Solid Edge part; units mm, degrees
sketch "Sketch1" plane through (0, 0, 0) normal (0, -1, 0) x (1, 0, 0)
  line L0 (0.9, 0.9) -> (0.9, 2.2249)
  arc A0 (-0.9, 2.2249) -> (0.9, 2.2249) centre (0, 0) cw
  line L1 (-0.9, 0.9) -> (-0.9, 2.2249)
  line L2 (-0.9, 0.9) -> (-2.2249, 0.9)
  line L3 (-0.9, -0.9) -> (-2.2249, -0.9)
  line L4 (-0.9, -0.9) -> (-0.9, -2.2249)
  arc A1 (0.9, -2.2249) -> (-0.9, -2.2249) centre (0, 0) cw
  line L5 (0.9, -0.9) -> (0.9, -2.2249)
  line L6 (0.9, -0.9) -> (2.2249, -0.9)
  arc A2 (2.2249, 0.9) -> (2.2249, -0.9) centre (0, 0) cw
  line L7 (0.9, 0.9) -> (2.2249, 0.9)
  arc A3 (-2.2249, 0.9) -> (-2.2249, -0.9) centre (0, 0) ccw
  line L8 (1.5624, 3.2433) -> (1.8936, 2.4029)
  line L9 (1.8936, 2.4029) -> (2.4029, 1.8936)
  line L10 (3.2433, 1.5624) -> (2.4029, 1.8936)
  arc A4 (3.2433, 1.5624) -> (3.2433, -1.5624) centre (0, 0) cw
  line L11 (2.4029, -1.8936) -> (3.2433, -1.5624)
  line L12 (2.4029, -1.8936) -> (1.8936, -2.4029)
  line L13 (1.5624, -3.2433) -> (1.8936, -2.4029)
  line L14 (-1.5624, -3.2433) -> (-1.8936, -2.4029)
  line L15 (-2.4029, -1.8936) -> (-1.8936, -2.4029)
  line L16 (-3.2433, -1.5624) -> (-2.4029, -1.8936)
  arc A5 (-3.2433, -1.5624) -> (-3.2433, 1.5624) centre (0, 0) cw
  line L17 (-3.2433, 1.5624) -> (-2.4029, 1.8936)
  line L18 (-2.4029, 1.8936) -> (-1.8936, 2.4029)
  line L19 (-1.8936, 2.4029) -> (-1.5624, 3.2433)
  arc A6 (-1.5624, 3.2433) -> (1.5624, 3.2433) centre (0, 0) cw
  arc A7 (1.5624, -3.2433) -> (-1.5624, -3.2433) centre (0, 0) cw
extrude "Protrusion1" add sketch "Sketch1" against normal blind 16
fillet "Round_1" radius 0.5 4 edges at (-0.9, 8, 0.9) (0.9, 8, 0.9) (-0.9, 8, -0.9) (0.9, 8, -0.9)
fillet "Round_2" radius 0.1 8 edges at (-0.9, 8, 2.2249) (0.9, 8, 2.2249) (2.2249, 8, 0.9) (2.2249, 8, -0.9) (0.9, 8, -2.2249) (-0.9, 8, -2.2249) (-2.2249, 8, -0.9) (-2.2249, 8, 0.9)
Geometry check sheet. Reference: the model listing, model coordinates, mm. A direction names the side the tool comes from. Give positions to 0.01 mm unless a question says otherwise; leave off trailing zeros. Write each loop counter-clockwise with the first axis right and the second up, starting at its lowest first coordinate (ties: lowest second). Pieces come first, ordered by that corner, then holes. Notation, with made-up numbers: M 19,61 L 51,61 A13 ccw 51,85 Z; hole C 8.5,58.25 d3. An arc over 180 degrees is marked long. Answer as CSV lines item,"result". Start each with the question number.
Q1. Release check for a two-part mould opening along Z. For faces 3 (the face through (-1.726, 7.888, -2.829)), 4 (the face through (-2, 16, 2)), 5 (the face through (0, 7.9, -2.4)) record: pulls with the +Z half, pulls with the -Z half, needs draft (parallel to the pull), parting line crosses it, or undercut.
Q2. Section check A-A, the plane z = -0.5. Record the cut outline in (x, y), then the cut area to 3 significant figures.
Q3. Section check B-B, the plane x = 0.25. Record the cut outline in (y, z).
Q4. Material ranges on L1, parallel to X at y = 15, z = -1.25; L2, parallel to Z at x = 2, y = 10.25, recorded low to high.
Q5. Section check C-C, the plane z = -3. Record the cut outline in (x, y).
Q6. Tool access check on faces 1 (the face through (2.82, 7.89, -1.73)), 2 (the face through (0, 7.9, 2.4)). Record the directions out of +Z, -Z, +X, -X, +Y, -Y that give a thin tool (end or side, any length) a straight path to the whole face; none if there is none.
Q7. Go/stop test with flat-tipped pins: pin 1 (0.8 mm diameter, centred on x = -1.5, y = 8, fed in from -Z); pin 2 (0.6 mm diameter, centred on y = 11.5, z = -1.5, fed in from +X); pin 3 (4 mm diameter, centred on y = 9, z = -2.5, fed in from -X). Record where each tip stops, or that it passes through.
Geometry says:
1,face 3,"pulls with the -Z half"
1,face 4,"needs draft"
1,face 5,"undercut"
2,outline,"M -3.57,0 L -2.35,0 L -2.35,16 L -3.57,16 Z; M 2.35,0 L 3.57,0 L 3.57,16 L 2.35,16 Z"
2,area,"39.0 mm^2"
3,outline,"M 0,-3.59 L 16,-3.59 L 16,-2.39 L 0,-2.39 Z; M 0,2.39 L 16,2.39 L 16,3.59 L 0,3.59 Z"
4,L1,"-3.38 to -0.92, 0.92 to 3.38"
4,L2,"-2.3 to -0.9, 0.9 to 2.3"
5,outline,"M -1.66,0 L 1.66,0 L 1.66,16 L -1.66,16 Z"
6,face 1,"-Z, +X, +Y, -Y"
6,face 2,"+Y, -Y"
7,pin 1,"z = -3.43"
7,pin 2,"x = 3.39"
7,pin 3,"x = -3.57"
